Verification items for the finished model (mm, model axes). Face numbers are marked on the shaded views. A direction names the side the tool comes from. Round coordinates to 2 decimals unless told otherwise and drop trailing zeros. Loops run counter-clockwise (first coordinate to the right, second up) from the corner with the lowest first, then second, coordinate; pieces in that order, holes last.
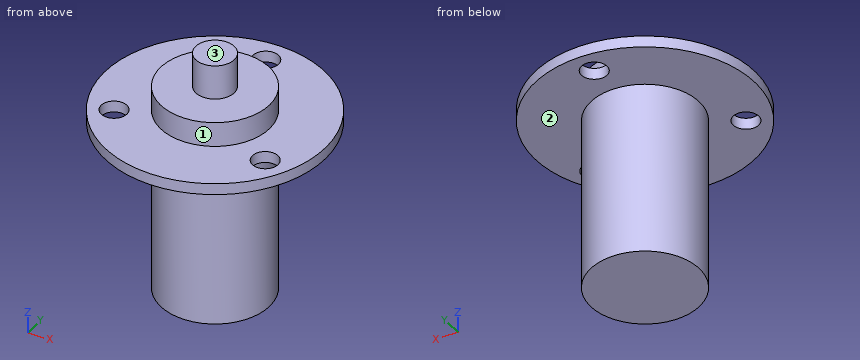
from build123d import *

# Parameters (mm, degrees)
BOSS_EXTRUDE1_DEPTH      = 5
BOSS_EXTRUDE1_DEPTH_BACK = 37.5
SKETCH1_R                = 11
SKETCH1_R_2              = 3.9
SKETCH1_3_R              = 22.25
SKETCH1_3_R_2            = 2.6
SKETCH1_3_R_3            = 11
BOSS_EXTRUDE2_DEPTH      = 2.3
BOSS_EXTRUDE4_DEPTH      = 12
BOSS_EXTRUDE4_DEPTH_BACK = 37.5
SKETCH1_4_R              = 3.9


with BuildPart() as part:
    # Sketch1 → Boss-Extrude1 (new, two sides: drawn at the far end of the back side and taken through both)
    with BuildSketch(Plane.XY.offset(-BOSS_EXTRUDE1_DEPTH_BACK)):
        Circle(SKETCH1_R)
        Circle(SKETCH1_R_2, mode=Mode.SUBTRACT)
    extrude(amount=BOSS_EXTRUDE1_DEPTH + BOSS_EXTRUDE1_DEPTH_BACK)

    # Sketch1<3> → Boss-Extrude2 (add)
    with BuildSketch(Plane.XY):
        Circle(SKETCH1_3_R)
        with Locations((-15.112143296, -8.725)):
            Circle(SKETCH1_3_R_2, mode=Mode.SUBTRACT)
        with Locations((15.112143296, -8.725)):
            Circle(SKETCH1_3_R_2, mode=Mode.SUBTRACT)
        with Locations((0, 17.45)):
            Circle(SKETCH1_3_R_2, mode=Mode.SUBTRACT)
        Circle(SKETCH1_3_R_3, mode=Mode.SUBTRACT)
    extrude(amount=-BOSS_EXTRUDE2_DEPTH)

    # Sketch1<4> → Boss-Extrude4 (add, two sides: drawn at the far end of the back side and taken through both)
    with BuildSketch(Plane.XY.offset(-BOSS_EXTRUDE4_DEPTH_BACK)):
        Circle(SKETCH1_4_R)
    extrude(amount=BOSS_EXTRUDE4_DEPTH + BOSS_EXTRUDE4_DEPTH_BACK)


solid = part.part
1. Section check A-A (x = 0). Enter the section's corners in (y, z).
2. Section check D-D (z = -18). Enter the section's corners in (x, y), then the cut area to 3 significant figures.
3. Tool access check on the marked faces 1, 2 and 3. Record the directions out of +Z, -Z, +X, -X, +Y, -Y that give a thin tool (end or side, any length) a straight path to the whole face; none if there is none.
4. Section check C-C (y = 17.45). Enter the section's corners in (x, z).
5. Gauge pin test, flat ends, axial feed: P1, Ø6, axis at x = 15.11, y = -8.72, coming from the -Z side; P2, Ø8.5, axis at x = -15.11, y = -8.72, coming from the +Z side; P3, Ø8, axis at x = 14.5, y = 1, coming from the +Z side; P4, Ø5, axis at y = 15, z = -22.5, coming from the +X side. Record the tip position at first contact, or that the pin passes through.
6. Scan lines: L1, parallel to Y at x = 0, z = -1.1; L2, parallel to Z at x = -1, y = -9; L3, parallel to Z at x = -14, y = -1. Record each from-to range of solid material in increasing order.
7. Section check B-B (y = 0). Enter the section's corners in (x, z).
Taken from the geometry:
1. outline: (-22.25, -2.3) - (-11, -2.3) - (-11, -37.5) - (11, -37.5) - (11, -2.3) - (14.85, -2.3) - (14.85, 0) - (11, 0) - (11, 5) - (3.9, 5) - (3.9, 12) - (-3.9, 12) - (-3.9, 5) - (-11, 5) - (-11, 0) - (-22.25, 0) - close; (20.05, -2.3) - (22.25, -2.3) - (22.25, 0) - (20.05, 0) - close
2. outline: circle Ø22 at (0, 0)
2. area: 380 mm2
3. face 1: +Z
3. face 2: -Z
3. face 3: +Z, +X, -X, +Y, -Y
4. outline: (-13.8, -2.3) - (-2.6, -2.3) - (-2.6, 0) - (-13.8, 0) - close; (2.6, -2.3) - (13.8, -2.3) - (13.8, 0) - (2.6, 0) - close
5. P1: stops at z = -2.3
5. P2: stops at z = 0
5. P3: stops at z = 5
5. P4: passes through
6. L1: y = -22.25 to 14.85, 20.05 to 22.25
6. L2: z = -37.5 to 5
6. L3: z = -2.3 to 0
7. outline: (-22.25, -2.3) - (-11, -2.3) - (-11, -37.5) - (11, -37.5) - (11, -2.3) - (22.25, -2.3) - (22.25, 0) - (11, 0) - (11, 5) - (3.9, 5) - (3.9, 12) - (-3.9, 12) - (-3.9, 5) - (-11, 5) - (-11, 0) - (-22.25, 0) - close
